```python
from build123d import *

# Parameters (mm, degrees)
SKETCH_3_R = 0.423054932
SKETCH_5_R = 0.423054932


with BuildPart() as part:
    # Эскиз1 → Повернуть2 (revolve)
    with BuildSketch(Plane(origin=(0, 0, 0), x_dir=(1, 0, 0), z_dir=(0, 1, 0))):
        with BuildLine():
            ThreePointArc((-1.749578385, 0.423054932), (0, 1.8), (1.749578385, 0.423054932))
            Line((1.749578385, 0.423054932), (1.749578385, 0))
            Line((1.749578385, 0), (-1.749578385, 0))
            Line((-1.749578385, 0), (-1.749578385, 0.423054932))
        make_face()
    revolve(axis=Axis((-29.751182373, 0, 0), (1, 0, 0)))

    # По траектории1: sweep along a path in Эскиз2
    with BuildLine(Plane.XY) as sweep_1_path:
        Line((-0.817553267, 0), (-5.35, 0))
        ThreePointArc((-5.35, 0), (-6.057106781, -0.292893219), (-6.35, -1))
        Line((-6.35, -1), (-6.35, -11.514871198))
    # Эскиз3 → По траектории1 (sweep)
    with BuildSketch(Plane.ZY.offset(1.749578385)):
        Circle(SKETCH_3_R)
    sweep(path=sweep_1_path.line)

    # По траектории2: sweep along a path in Эскиз4
    with BuildLine(Plane.XY) as sweep_2_path:
        Line((6.35, -11.514871198), (6.35, -1))
        ThreePointArc((6.35, -1), (6.057106781, -0.292893219), (5.35, 0))
        Line((5.35, 0), (0.821594736, 0))
    # Эскиз5 → По траектории2 (sweep)
    with BuildSketch(Plane(origin=(1.749578385, 0, 0), x_dir=(0, 0, -1), z_dir=(1, 0, 0))):
        Circle(SKETCH_5_R)
    sweep(path=sweep_2_path.line)


solid = part.part
```
Input: part model. Units: mm. Frame: model coordinates. A direction names the side the tool comes from. Round coordinates to 2 decimals unless told otherwise and drop trailing zeros. Order: outer loops, then holes, each group sorted by start corner. A loop starts at its lowest first (then second) coordinate and runs counter-clockwise, first axis right, second up. Notation, with made-up numbers: (29.5, 64) - (78.5, 64) arc R15 cw to (78.5, 68) - close; hole circle Ø6 at (0, 78). An arc over 180 degrees is marked (long way). One line per question, with ' | ' between items. Start each with the question number.
1) Ray query, probe 1 along X at (y, z) = (-9.5, -0.25); probe 2 along X at (y, z) = (-4.25, -0.3); probe 3 along Y at (x, z) = (-0.25, -1.2). Return the intervals inside material, ascending.
2) Pull-direction query (X, two-part tool) for faces 1 (the cylindrical face through (6.763, -6.184, 0.092)), 2 (the flat face through (-6.3, -11.515, 0)); classes: +X half, -X half, draft (parallel to the pull), parting line (faces both ways), or undercut.
3) Cut plane C-C, the plane x = -4. Return the cut outline in (y, z).
4) Set-up query: faces 3 (the cylindrical face through (-5.937, -6.331, -0.092)), 4 (the flat face through (6.4, -11.515, 0)), 5 (the cylindrical face through (3.5, -0.3, 0.3)). Return all of +Z, -Z, +X, -X, +Y, -Y with unobstructed straight access to the full face (end or side cutting, diameter ignored); none if empty.
5) Cut plane B-B, the plane z = 0.2. Return the cut outline in (x, y), then the cut area to 3 significant figures.
6) Cut plane A-A, the plane y = -3. Return the cut outline in (x, z).
7) Contact query for flat-ended pins moving along their axis: P1, Ø1, axis at y = -0.5, z = 1.5, coming from the -X side; P2, Ø1.5, axis at x = 3.5, z = 1, coming from the +Y side; P3, Ø1.5, axis at y = -2.5, z = 1, coming from the -X side. Output: stop coordinate, or through.
8) Cut plane D-D, the plane y = -0.75. Give the number of separate pieces and of enclosed holes in the cut face, then the cut area to 3 significant figures.
Worked out:
1) probe 1: x = -6.69 to -6.01, 6.01 to 6.69 | probe 2: x = -6.65 to -6.05, 6.05 to 6.65 | probe 3: y = -1.32 to 1.32
2) face 1: undercut | face 2: draft
3) outline: circle Ø0.85 at (0, 0)
4) face 3: -Y | face 4: +Z, -Z, +X, -X, -Y | face 5: none
5) outline: (-6.72, -11.51) - (-5.98, -11.51) - (-5.98, -1) arc R0.63 cw to (-5.35, -0.37) - (-1.75, -0.37) arc R1.79 ccw to (1.75, -0.37) - (5.35, -0.37) arc R0.63 cw to (5.98, -1) - (5.98, -11.51) - (6.72, -11.51) - (6.72, -1) arc R1.37 ccw to (5.35, 0.37) - (1.75, 0.37) arc R1.79 ccw to (-1.75, 0.37) - (-5.35, 0.37) arc R1.37 ccw to (-6.72, -1) - close | area: 33.4 mm^2
6) outline: circle Ø0.85 at (-6.35, 0); circle Ø0.85 at (6.35, 0)
7) P1: stops at x = -1.44 | P2: stops at y = 0.34 | P3: stops at x = -6.69
8) separate pieces: 3 | enclosed holes: 0 | area: 9.58 mm^2
